Could you check a few things on this model? Use its own coordinates, in mm. A direction names the side the tool comes from. Coordinates: 2 decimals unless noted, no trailing zeros. Loops run counter-clockwise (first coordinate to the right, second up) from the corner with the lowest first, then second, coordinate; pieces in that order, holes last.
1) If I drill on line 1 along X through (y, z) = (1.6, -62.5); line 2 along Z through (x, y) = (32, 0.65); line 3 along X through (y, z) = (3.35, -94.5), over which ranges is the centre line in solid material (lowest first)?
2) For faces 1 (the face through (35, 3, -60.393)), 2 (the face through (38, 2, 89.393)), 3 (the face through (20, 2, -95)), which set-ups out of +Z, -Z, +X, -X, +Y, -Y let a thin tool reach every point of the face, with its end or its side?
3) Thinking about a two-plate mould opening in Z: for faces 4 (the face through (6.879, 2.465, 97.247)), 5 (the face through (38, 2, -89.393)), 6 (the face through (8, 2, 100)), 7 (the face through (7.121, 2.465, -97.247)), which applies, released by +Z, released by -Z, zero draft, split by the parting line, or undercut?
4) Imagine slicing it at B-B on y = 2.6. Please give me the cut outline in (x, z), plus the area to 4 significant figures.
5) Imagine slicing it at D-D on z = -62.5. Please give me the cut outline in (x, y), plus the area to 3 significant figures.
6) Will these pins go through, and if not, where does the flat tip stop? P1, Ø2.5, axis at x = 42, y = 1.5, coming from the +Z side; P2, Ø1.5, axis at x = 32.5, y = 2, coming from the -Z side; P3, Ø1.5, axis at x = 22, y = 3, coming from the -Z side.
7) Imagine slicing it at A-A on z = -94.5. Please give me the cut outline in (x, y).
8) Imagine slicing it at C-C on x = 7. Please give me the cut outline in (y, z), plus the area to 3 significant figures.
```python
from build123d import *

# Parameters (mm, degrees)
ESQUISSE1_R             = 2.75
BOSS_EXTRU_1_DEPTH      = 5
ESQUISSE2_W             = 30
ESQUISSE2_H             = 15
ENL_V_MAT_EXTRU_1_DEPTH = 112.915146428


with BuildPart() as part:
    # Esquisse1 → Boss.-Extru.1 (new body)
    with BuildSketch(Plane(origin=(0, 0, 0), x_dir=(1, 0, 0), z_dir=(0, 1, 0))):
        Polygon((0, 100), (15, 100), (25.606601718, 89.393398282), (50, 89.393398282), (50, -89.393398282), (25.606601718, -89.393398282), (15, -100), (0, -100), align=None)
        with Locations(Location((7, 94.5, 0), (0, 0, 270))):
            Circle(ESQUISSE1_R, mode=Mode.SUBTRACT)
        with Locations(Location((7, 62.5, 0), (0, 0, 270))):
            Circle(ESQUISSE1_R, mode=Mode.SUBTRACT)
        with Locations(Location((7, -62.5, 0), (0, 0, 90))):
            Circle(ESQUISSE1_R, mode=Mode.SUBTRACT)
        with Locations(Location((7, -94.5, 0), (0, 0, 90))):
            Circle(ESQUISSE1_R, mode=Mode.SUBTRACT)
    extrude(amount=BOSS_EXTRU_1_DEPTH)

    # Esquisse2 → Enlèv. mat.-Extru.1 (cut, through all)
    with BuildSketch(Plane(origin=(0, 5, 0), x_dir=(1, 0, 0), z_dir=(0, 1, 0))):
        with Locations((35, 67.893398282)):
            Rectangle(ESQUISSE2_W, ESQUISSE2_H)
    extrude(amount=-ENL_V_MAT_EXTRU_1_DEPTH, mode=Mode.SUBTRACT)


solid = part.part
```
Filled in:
1. line 1: x = 0 to 4.25, 9.75 to 20
1. line 2: z = -89.39 to -75.39, -60.39 to 89.39
1. line 3: x = 0 to 4.25, 9.75 to 20.5
2. face 1: +X, +Y, -Y
2. face 2: +Z, +X, +Y, -Y
2. face 3: -Z, +X, +Y, -Y
3. face 4: undercut
3. face 5: released by -Z
3. face 6: released by +Z
3. face 7: undercut
4. outline: (0, -100) - (15, -100) - (25.61, -89.39) - (50, -89.39) - (50, -75.39) - (20, -75.39) - (20, -60.39) - (50, -60.39) - (50, 89.39) - (25.61, 89.39) - (15, 100) - (0, 100) - close; hole circle Ø5.5 at (7, -94.5); hole circle Ø5.5 at (7, -62.5); hole circle Ø5.5 at (7, 62.5); hole circle Ø5.5 at (7, 94.5)
4. area: 8,825 mm2
5. outline: (0, 0) - (4.25, 0) - (4.25, 5) - (0, 5) - close; (9.75, 0) - (20, 0) - (20, 5) - (9.75, 5) - close
5. area: 72.5 mm2
6. P1: stops at z = 89.39
6. P2: stops at z = -89.39
6. P3: stops at z = -93.75
7. outline: (0, 0) - (4.25, 0) - (4.25, 5) - (0, 5) - close; (9.75, 0) - (20.5, 0) - (20.5, 5) - (9.75, 5) - close
8. outline: (0, -100) - (5, -100) - (5, -97.25) - (0, -97.25) - close; (0, -91.75) - (5, -91.75) - (5, -65.25) - (0, -65.25) - close; (0, -59.75) - (5, -59.75) - (5, 59.75) - (0, 59.75) - close; (0, 65.25) - (5, 65.25) - (5, 91.75) - (0, 91.75) - close; (0, 97.25) - (5, 97.25) - (5, 100) - (0, 100) - close
8. area: 890 mm2
